from build123d import *
from build123d import SkipClean  # not in build123d's __all__

# Parameters (mm, degrees)
F0_R      = 2.5
F1_DEPTH  = 15
F3_DEPTH  = 29
F4_R      = 1.5
F5_DEPTH  = 7.15
F6_R      = 1
F7_DEPTH  = 7.15
F10_DEPTH = 55


with BuildPart() as f1:
    # F0 (on Top) → F1 (new body)
    with BuildSketch(Plane.XY):
        with BuildLine():
            Line((0, 0), (-20, 0))
            Line((-20, 0), (-41.2132034356, -21.2132034356))
            Line((-41.2132034356, -21.2132034356), (-20.7071067812, -41.71930009))
            Line((-20.7071067812, -41.71930009), (-6.5649711575, -27.5771644663))
            Line((-6.5649711575, -27.5771644663), (0, -27.5771644663))
            Line((0, -27.5771644663), (0, -25.0771644663))
            ThreePointArc((0, -25.0771644663), (-2.5, -22.5771644663), (0, -20.0771644663))
            Line((0, -20.0771644663), (0, 0))
        make_face()
        with Locations((-15, -5)):
            Circle(F0_R, mode=Mode.SUBTRACT)
    extrude(amount=F1_DEPTH)

    # F2 (on face) → F3 (cut, through all)
    with BuildSketch(Plane(origin=(-10, 10, 0), x_dir=(-0.7071067812, -0.7071067812, 0), z_dir=(-0.7071067812, 0.7071067812, 0))):
        with BuildLine():
            Line((44.1421356237, 7.85), (36.8814735646, 7.85))
            ThreePointArc((36.8814735646, 7.85), (25.3921356237, 7.5), (36.8814735646, 7.15))
            Line((36.8814735646, 7.15), (44.1421356237, 7.15))
            Line((44.1421356237, 7.15), (44.1421356237, 7.85))
        make_face()
    extrude(amount=-F3_DEPTH, mode=Mode.SUBTRACT)

    # F4 (on face) → F5 (cut, through all)
    with BuildSketch(Plane.XY.offset(15)):
        with Locations((-34.1421356237, -22.627416998)):
            Circle(F4_R)
        with Locations((-22.1213203436, -34.6482322781)):
            Circle(F4_R)
    extrude(amount=-F5_DEPTH, mode=Mode.SUBTRACT)

    # F6 (on face) → F7 (cut, through all)
    with BuildSketch(Plane(origin=(0, 0, 0), x_dir=(1, 0, 0), z_dir=(0, 0, -1))):
        with Locations((-22.1213203436, 34.6482322781)):
            Circle(F6_R)
        with Locations((-34.1421356237, 22.627416998)):
            Circle(F6_R)
    extrude(amount=-F7_DEPTH, mode=Mode.SUBTRACT)

    # F8: F1 across plane


with BuildPart() as f1_1:
    add(f1.part, clean=False)
    with SkipClean():  # cleaning this boolean's faces spoils the solid; the shape is the same uncleaned
        add(f1.part.mirror(Plane.YZ), clean=False)

    # F9 (on face) → F10 (cut)
    with BuildSketch(Plane(origin=(0, 0, 0), x_dir=(-1, 0, 0), z_dir=(0, 1, 0))):
        Polygon((47.4618822336, 7.5), (-20, 7.5), (-48.8657653332, 7.5), (-48.8657653332, -7.0414701477), (47.4618822336, -7.0414701477), align=None)
    with SkipClean():  # cleaning this boolean's faces spoils the solid; the shape is the same uncleaned
        extrude(amount=-F10_DEPTH, mode=Mode.SUBTRACT)


solid = f1_1.part
Read the model definition and answer for the solid it produces. Units are mm, in the model's axes. A direction names the side the tool comes from. Coordinates: 2 decimals unless noted, no trailing zeros. Loops run counter-clockwise (first coordinate to the right, second up) from the corner with the lowest first, then second, coordinate; pieces in that order, holes last. Notation, with made-up numbers: (27.5, -6.5) -> (68.5, -6.5) arc R23 cw to (68.5, 10.5) -> close; hole circle Ø9 at (-19, 76.25). An arc over 180 degrees is marked (long way). Answer in a Markdown table with one row per item.
Item 1: A cutting plane is placed at A-A on z = 12. Give the number of separate pieces and of enclosed holes in the cut face, plus the area to 3 significant figures.
Returned:
| item | result |
|---|---|
| separate pieces | 3 |
| enclosed holes | 7 |
| area | 1,680 mm^2 |
Item 2: Straight lines are drawn through the part: line 1 along X through (y, z) = (-36, 14); line 2 along X through (y, z) = (-4, 11.5); line 3 along X through (y, z) = (-21.5, 11.25). For each, find the intervals that lie inside material, in ascending order. Write a range as [from, to].
Returned:
| item | result |
|---|---|
| line 1 | x = [-26.43, -22.77], [-21.47, -14.99], [14.99, 21.47], [22.77, 26.43] |
| line 2 | x = [-24, -17.29], [-12.71, 12.71], [17.29, 24] |
| line 3 | x = [-40.93, -35.13], [-33.15, -28.71], [-16.38, -2.26], [2.26, 16.38], [28.71, 33.15], [35.13, 40.93] |
Item 3: For faces 5 (the flat face through (31.104, -31.323, 11.375)), 6 (the flat face through (0, -27.577, 11)), 7 (the flat face through (29, -29, 7.85)), 8 (the flat face through (-29, -29, 7.85)), determine the directions among +Z, -Z, +X, -X, +Y, -Y from which every point of the face is accessible in a straight line to the end or side of a thin tool.
Returned:
| item | result |
|---|---|
| face 5 | +Z, -Z, +X, -Y |
| face 6 | +Z, -Z, -Y |
| face 7 | -Z, +X, -Y |
| face 8 | -Z, -X, -Y |
Item 4: A cutting plane is placed at B-B on y = -5. Determine the outline of the cut face in (x, z), plus the area to 3 significant figures.
Returned:
| item | result |
|---|---|
| outline | (-25, 7.5) -> (-17.5, 7.5) -> (-17.5, 15) -> (-25, 15) -> close; (-12.5, 7.5) -> (12.5, 7.5) -> (12.5, 15) -> (-12.5, 15) -> close; (17.5, 7.5) -> (25, 7.5) -> (25, 15) -> (17.5, 15) -> close |
| area | 300 mm^2 |
Item 5: Each of these flat-tipped pins is pushed along its axis until it touches: P1, Ø7.5, axis at x = -24.5, y = -28.5, coming from the -Z side; P2, Ø2, axis at x = 1.5, z = 9.5, coming from the -Y side; P3, Ø1.5, axis at y = -24.5, z = 11, coming from the +X side. Where does it stop, or does it pass through?
Returned:
| item | result |
|---|---|
| P1 | stops at z = 7.85 |
| P2 | stops at y = -27.58 |
| P3 | stops at x = 38.68 |
Item 6: For a pull along X with two mould halves and no side action, classify faces 1 (the cylindrical face through (-21.88, -22.09, 13.25)), 2 (the flat face through (30, -10, 13)), 3 (the flat face through (-31.104, -31.323, 11.375)), 4 (the flat face through (1, -16, 15)) as released by +X, released by -X, zero draft, split by the parting line, or undercut.
Returned:
| item | result |
|---|---|
| face 1 | undercut |
| face 2 | released by +X |
| face 3 | released by -X |
| face 4 | zero draft |
